from build123d import *

# Parameters (mm, degrees)
SKETCH2_R           = 3.3
SKETCH2_R_2         = 3
BOSS_EXTRUDE1_DEPTH = 4
CUT_EXTRUDE1_DEPTH  = 5


with BuildPart() as part:
    # Sketch2 → Boss-Extrude1 (new body)
    with BuildSketch(Plane.XY):
        Circle(SKETCH2_R)
        Circle(SKETCH2_R_2, mode=Mode.SUBTRACT)
    extrude(amount=BOSS_EXTRUDE1_DEPTH)

    # Sketch3 → Cut-Extrude1 (cut)
    with BuildSketch(Plane(origin=(0, 3.3, 0), x_dir=(1, 0, 0), z_dir=(0, 1, 0))):
        Polygon((1.85, -4), (2.35, -4), (2.35, -2.60176001), (-1.85, -1.4), (-1.85, 0), (-2.35, 0), (-2.35, -1.4), (1.85, -2.60176001), align=None)
    extrude(amount=-CUT_EXTRUDE1_DEPTH, mode=Mode.SUBTRACT)


solid = part.part
Could you check a few things on this model? Use its own coordinates, in mm. Give positions to 0.01 mm unless a question says otherwise; leave off trailing zeros. Order: outer loops, then holes, each group sorted by start corner. A loop starts at its lowest first (then second) coordinate and runs counter-clockwise, first axis right, second up.
Item 1: I'm going to push a flat-ended pin straight in: pin 1 (2 mm diameter, centred on x = -2.5, z = 1, fed in from +Y). Where does the tip first touch, or does it pass through?
Item 2: If we section it at D-D, the plane z = 0.4: Write out the boundary of the cut face in (x, y).
Item 3: If we section it at A-A, the plane x = 0.25: Write out the boundary of the cut face in (y, z).
Item 4: If we section it at C-C, the plane x = 2.75: Write out the boundary of the cut face in (y, z), plus the area to 3 significant figures.
Item 5: I need wall thicknesses on line 1 (X direction, y = 0, z = 1.75); line 2 (Y direction, x = 1.75, z = 3.55). Which ranges of each line are inside material? Lowest first, please.
Item 6: If we section it at B-B, the plane y = 1.25: Write out the boundary of the cut face in (x, z).
Values:
1. pin 1: stops at y = 2.94
2. outline: (-2.35, 1.86) - (-2.35, 2.32) arc R3.3 ccw (long way) to (-1.85, 2.73) - (-1.85, 2.36) arc R3 cw (long way) to start
3. outline: (-3.29, 0) - (-2.99, 0) - (-2.99, 4) - (-3.29, 4) - close; (2.99, 0) - (3.29, 0) - (3.29, 2) - (2.99, 2) - close; (2.99, 2.14) - (3.29, 2.14) - (3.29, 4) - (2.99, 4) - close
4. outline: (-1.82, 0) - (-1.2, 0) - (-1.2, 4) - (-1.82, 4) - close; (1.2, 0) - (1.82, 0) - (1.82, 4) - (1.2, 4) - close
4. area: 5.00 mm2
5. line 1: x = -3.3 to -3, 3 to 3.3
5. line 2: y = -2.8 to -2.44, 2.44 to 2.8
6. outline: (-3.05, 0) - (-2.73, 0) - (-2.73, 4) - (-3.05, 4) - close; (2.73, 0) - (3.05, 0) - (3.05, 4) - (2.73, 4) - close
